```python
from build123d import *

# Parameters (mm, degrees)
SKETCH1_W                                      = 50.8
SKETCH1_H                                      = 12.7
BOSS_EXTRUDE1_DEPTH                            = 27.94
BOSS_EXTRUDE2_START                            = 27.94
SKETCH1_3_W                                    = 50.8
SKETCH1_3_H                                    = 12.7
BOSS_EXTRUDE2_DEPTH                            = 12.7
BOSS_EXTRUDE3_START                            = -40.64
SKETCH1_4_W                                    = 50.8
SKETCH1_4_H                                    = 12.7
BOSS_EXTRUDE3_DEPTH                            = 12.7
SKETCH2_R                                      = 9.525
CUT_EXTRUDE1_DEPTH                             = 115.271774293
RIB6_REACH                                     = 92.018
SKETCH4_WALL_W                                 = 217.956683174
SKETCH4_WALL_H                                 = 5.08
CBORE_START                                    = 8.509
CBORE_FOR_1_4_BINDING_HEAD_MACHINE_S_2_R       = 7.14375
CBORE_FOR_1_4_BINDING_HEAD_MACHINE_SCREW_DEPTH = 4.191
CBORE_FOR_1_4_BINDING_HEAD_MACHINE_S_3_O_R     = 3.3782
CBORE_FOR_1_4_BINDING_HEAD_MACHINE_S_3_DEPTH   = 8.509


# Read off the part's stored shape, not the designer's step: CBORE for 1/4 Binding Head Machine Screw1
with BuildPart() as part:
    # Sketch1 → Boss-Extrude1 (new, symmetric)
    with BuildSketch(Plane.XY):
        with Locations((0, 6.35)):
            Rectangle(SKETCH1_W, SKETCH1_H)
    extrude(amount=BOSS_EXTRUDE1_DEPTH, both=True)

    # Sketch1<3> → Boss-Extrude2 (add)
    with BuildSketch(Plane.XY.offset(BOSS_EXTRUDE2_START)):
        with BuildLine():
            Line((-25.4, 50.8), (-25.4, 12.7))
            Line((-25.4, 12.7), (25.4, 12.7))
            Line((25.4, 12.7), (25.4, 50.8))
            ThreePointArc((25.4, 50.8), (0, 76.2), (-25.4, 50.8))
        make_face()
        with Locations((0, 6.35)):
            Rectangle(SKETCH1_3_W, SKETCH1_3_H)
    extrude(amount=BOSS_EXTRUDE2_DEPTH)

    # Sketch1<4> → Boss-Extrude3 (add)
    with BuildSketch(Plane.XY.offset(BOSS_EXTRUDE3_START)):
        with BuildLine():
            Line((-25.4, 50.8), (-25.4, 12.7))
            Line((-25.4, 12.7), (25.4, 12.7))
            Line((25.4, 12.7), (25.4, 50.8))
            ThreePointArc((25.4, 50.8), (0, 76.2), (-25.4, 50.8))
        make_face()
        with Locations((0, 6.35)):
            Rectangle(SKETCH1_4_W, SKETCH1_4_H)
    extrude(amount=BOSS_EXTRUDE3_DEPTH)

    # Sketch2 → Cut-Extrude1 (cut, through all)
    with BuildSketch(Plane.XY.offset(40.64)):
        with Locations((0, 50.8)):
            Circle(SKETCH2_R)
    extrude(amount=-CUT_EXTRUDE1_DEPTH, mode=Mode.SUBTRACT)

    # Sketch4 wall → Rib6 (add, up to next)
    with BuildSketch(Plane(origin=(0, 25.4, 15.24), x_dir=(0, -0.707106781187, -0.707106781187), z_dir=(0, 0.707106781187, -0.707106781187)), mode=Mode.PRIVATE) as rib6_sk1:
        Rectangle(SKETCH4_WALL_W, SKETCH4_WALL_H)
    rib6_tool1 = extrude(rib6_sk1.sketch, amount=-RIB6_REACH, mode=Mode.PRIVATE) - part.part
    rib6 = rib6_tool1.solids().sort_by_distance((0, 25.4, 15.24))[0]
    add(rib6)

    # Mirror1: Rib6 across plane
    add(rib6.mirror(Plane.XY))

    # CBORE for 1_4 Binding Head Machine S 2 → CBORE for 1/4 Binding Head Machine Screw1 (cut)
    with BuildSketch(Plane(origin=(0, 0, 0), x_dir=(1, 0, 0), z_dir=(0, 1, 0)).offset(CBORE_START)):
        with Locations((12.7, -15.24)):
            Circle(CBORE_FOR_1_4_BINDING_HEAD_MACHINE_S_2_R)
        with Locations((12.7, 15.24)):
            Circle(CBORE_FOR_1_4_BINDING_HEAD_MACHINE_S_2_R)
        with Locations((-12.7, -15.24)):
            Circle(CBORE_FOR_1_4_BINDING_HEAD_MACHINE_S_2_R)
        with Locations((-12.7, 15.24)):
            Circle(CBORE_FOR_1_4_BINDING_HEAD_MACHINE_S_2_R)
    extrude(amount=CBORE_FOR_1_4_BINDING_HEAD_MACHINE_SCREW_DEPTH, mode=Mode.SUBTRACT)

    # CBORE for 1_4 Binding Head Machine S 3 o → CBORE for 1_4 Binding Head Machine S 3 (cut)
    with BuildSketch(Plane(origin=(0, 0, 0), x_dir=(1, 0, 0), z_dir=(0, 1, 0))):
        with Locations((12.7, -15.24)):
            Circle(CBORE_FOR_1_4_BINDING_HEAD_MACHINE_S_3_O_R)
        with Locations((12.7, 15.24)):
            Circle(CBORE_FOR_1_4_BINDING_HEAD_MACHINE_S_3_O_R)
        with Locations((-12.7, -15.24)):
            Circle(CBORE_FOR_1_4_BINDING_HEAD_MACHINE_S_3_O_R)
        with Locations((-12.7, 15.24)):
            Circle(CBORE_FOR_1_4_BINDING_HEAD_MACHINE_S_3_O_R)
    extrude(amount=CBORE_FOR_1_4_BINDING_HEAD_MACHINE_S_3_DEPTH, mode=Mode.SUBTRACT)


solid = part.part
```
Model file for the job. Use its own axes, mm. A direction names the side the tool comes from. Coordinates: 2 decimals unless noted, no trailing zeros. Order: outer loops, then holes, each group sorted by start corner. A loop starts at its lowest first (then second) coordinate and runs counter-clockwise, first axis right, second up. Notation, with made-up numbers: M 20,71 L 28,71 A23 cw 28,84 Z; hole C 20.25,-24.75 d7. An arc over 180 degrees is marked long. Answer as CSV lines item,"result".
(1) Band-saw the part on D-D, the plane y = 55. List the corners of the cut face in (x, z).
Geometry says:
outline,"M -25.05,-40.64 L -8.55,-40.64 L -8.55,-27.94 L -25.05,-27.94 Z; M -25.05,27.94 L -8.55,27.94 L -8.55,40.64 L -25.05,40.64 Z; M 8.55,-40.64 L 25.05,-40.64 L 25.05,-27.94 L 8.55,-27.94 Z; M 8.55,27.94 L 25.05,27.94 L 25.05,40.64 L 8.55,40.64 Z"
(2) Band-saw the part on B-B, the plane x = 12.7. List the corners of the cut face in (y, z), then the cut area to 3 significant figures.
Geometry says:
outline,"M 0,-40.64 L 72.8,-40.64 L 72.8,-27.94 L 12.7,-27.94 L 12.7,-22.38 L 8.51,-22.38 L 8.51,-18.62 L 0,-18.62 Z; M 0,-11.86 L 8.51,-11.86 L 8.51,-8.1 L 12.7,-8.1 L 12.7,8.1 L 8.51,8.1 L 8.51,11.86 L 0,11.86 Z; M 0,18.62 L 8.51,18.62 L 8.51,22.38 L 12.7,22.38 L 12.7,27.94 L 72.8,27.94 L 72.8,40.64 L 0,40.64 Z"
area,"2,320 mm2"
(3) Wall check: line 1 along X through (y, z) = (11, 15); line 2 along Z through (x, y) = (-12.7, 4.75); line 3 along X through (y, z) = (6.25, -15.24). Give the ranges that are in metal, low to high.
Geometry says:
line 1,"x = -25.4 to -19.84, -5.56 to 5.56, 19.84 to 25.4"
line 2,"z = -40.64 to -18.62, -11.86 to 11.86, 18.62 to 40.64"
line 3,"x = -25.4 to -16.08, -9.32 to 9.32, 16.08 to 25.4"
(4) Flat gauge pins, fed straight in: pin 1 (20.5 mm diameter, centred on y = 26, z = 16.5, fed in from +X); pin 2 (12 mm diameter, centred on x = -18.5, z = -21.5, fed in from +Y); pin 3 (7 mm diameter, centred on x = 12.5, z = -13, fed in from +Y). Where does each tip first touch, or does it go through?
Geometry says:
pin 1,"stops at x = 2.54"
pin 2,"stops at y = 12.7"
pin 3,"stops at y = 8.51"
(5) 3-axis set-ups, long thin cutter, end or side, ignore diameter. For faces 4 (the flat face through (0, 39, -40.64)), 5 (the flat face through (-2.54, 21, -20)), 6 (the cylindrical face through (-14.249, 10.575, 22.214)), 7 (the flat face through (2.54, 21, -20)), 8 (the flat face through (-0.04, 25.58, -15.42)): which of +Z, -Z, +X, -X, +Y, -Y reach the whole face in a straight line?
Geometry says:
face 4,"-Z, +X, -X, +Y, -Y"
face 5,"-X, +Y"
face 6,"+Y"
face 7,"+X, +Y"
face 8,"+X, -X, +Y"
(6) Band-saw the part on C-C, the plane z = -15.24. List the corners of the cut face in (x, y), then the cut area to 3 significant figures.
Geometry says:
outline,"M -25.4,0 L -16.08,0 L -16.08,8.51 L -19.84,8.51 L -19.84,12.7 L -25.4,12.7 Z; M -9.32,0 L 9.32,0 L 9.32,8.51 L 5.56,8.51 L 5.56,12.7 L 2.54,12.7 L 2.54,25.4 L -2.54,25.4 L -2.54,12.7 L -5.56,12.7 L -5.56,8.51 L -9.32,8.51 Z; M 16.08,0 L 25.4,0 L 25.4,12.7 L 19.84,12.7 L 19.84,8.51 L 16.08,8.51 Z"
area,"475 mm2"
(7) Pull direction X, two halves, no side cores. Call faces 1 (the flat face through (-0.04, 25.58, 15.42)), 2 (the flat face through (25.4, 8, -1)), 3 (the cylindrical face through (-1.24, 60.244, 34.379)): +X half, -X half, draft (parallel to the pull), parting line (faces both ways), or undercut.
Geometry says:
face 1,"draft"
face 2,"+X half"
face 3,"undercut"
(8) Band-saw the part on A-A, the plane y = 21. List the corners of the cut face in (x, z).
Geometry says:
outline,"M -25.4,-40.64 L 25.4,-40.64 L 25.4,-27.94 L 2.54,-27.94 L 2.54,-10.84 L -2.54,-10.84 L -2.54,-27.94 L -25.4,-27.94 Z; M -25.4,27.94 L -2.54,27.94 L -2.54,10.84 L 2.54,10.84 L 2.54,27.94 L 25.4,27.94 L 25.4,40.64 L -25.4,40.64 Z"
